```python
from build123d import *

# Parameters (mm, degrees)
F1_DEPTH = 38.1
F2_W     = 31.75
F2_H     = 73.025
F3_DEPTH = 152.401
F4_R     = 2.54
F5_R     = 2.54
F6_R     = 6.35
F7_DEPTH = 25.4
F8_R     = 4.7625
F9_DEPTH = 38.101


with BuildPart() as f1:
    # F0 (on Right) → F1 (new body)
    with BuildSketch(Plane.YZ):
        with BuildLine():
            Line((-57.15, 76.2), (-76.2, 76.2))
            Line((-76.2, 76.2), (-76.2, -13.9112576244))
            Line((-76.2, -13.9112576244), (-50.8, -13.9112576244))
            ThreePointArc((-50.8, -13.9112576244), (-41.275, -23.4362576244), (-50.8, -32.9612576244))
            Line((-50.8, -32.9612576244), (-76.2, -32.9612576244))
            Line((-76.2, -32.9612576244), (-76.2, -76.2))
            Line((-76.2, -76.2), (-38.1, -76.2))
            Line((-38.1, -76.2), (-12.7, -63.5))
            Line((-12.7, -63.5), (-12.7, 19.05))
            Line((-12.7, 19.05), (-57.15, 76.2))
        make_face()
    extrude(amount=F1_DEPTH)

    # F2 (on face) → F3 (cut, through all)
    with BuildSketch(Plane.XY.offset(76.2)):
        with Locations((19.05, -36.5125)):
            Rectangle(F2_W, F2_H)
    extrude(amount=-F3_DEPTH, mode=Mode.SUBTRACT)

    # F4
    f4_edges = [f1.edges().sort_by_distance(p)[0] for p in [
        (3.175, -73.025, 31.144371),
        (34.925, -73.025, 31.144371),
        (34.925, -73.025, -54.580629),
        (3.175, -73.025, -54.580629),
    ]]
    fillet(f4_edges, radius=F4_R)

    # F5
    f5_edges = [f1.edges().sort_by_distance(p)[0] for p in [
        (38.1, -76.2, -54.580629),
        (0, -76.2, -54.580629),
        (0, -76.2, 31.144371),
        (38.1, -76.2, 31.144371),
    ]]
    fillet(f5_edges, radius=F5_R)

    # F6 (on face) → F7 (cut)
    with BuildSketch(Plane.XZ.offset(76.2)):
        with Locations((19.05, -52.0112576244)):
            Circle(F6_R)
    extrude(amount=-F7_DEPTH, mode=Mode.SUBTRACT)

    # F8 (on face) → F9 (cut, through all)
    with BuildSketch(Plane.YZ.offset(38.1)):
        with Locations((-60.96, 57.15)):
            Circle(F8_R)
    extrude(amount=-F9_DEPTH, mode=Mode.SUBTRACT)


solid = f1.part
```
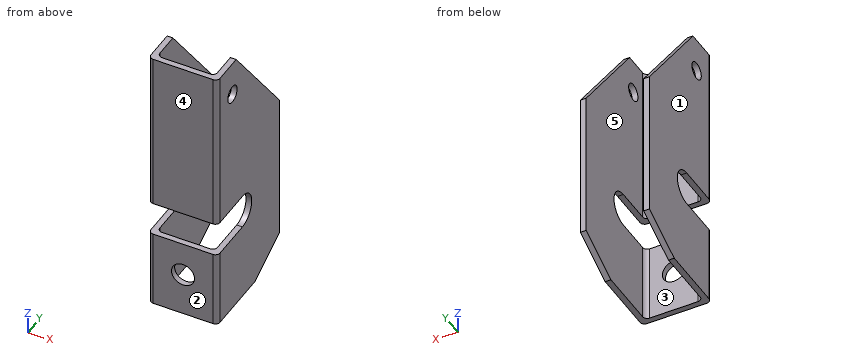
Input: part model. Units: mm. Frame: model coordinates. Face numbers are marked on the shaded views. A direction names the side the tool comes from. Give positions to 0.01 mm unless a question says otherwise; leave off trailing zeros. Order: outer loops, then holes, each group sorted by start corner. A loop starts at its lowest first (then second) coordinate and runs counter-clockwise, first axis right, second up.
1. Cut plane A-A (x = 19.05). Return loops of the section in (y, z) (3 decimals), and give its area (3 significant figures).
Computed:
outline: (-76.2, -76.2) - (-73.025, -76.2) - (-73.025, -58.361) - (-76.2, -58.361) - close; (-76.2, -45.661) - (-73.025, -45.661) - (-73.025, -32.961) - (-76.2, -32.961) - close; (-76.2, -13.911) - (-73.025, -13.911) - (-73.025, 76.2) - (-76.2, 76.2) - close
area: 383 mm2
2. Set-up query: the marked faces 4 and 5. Return all of +Z, -Z, +X, -X, +Y, -Y with unobstructed straight access to the full face (end or side cutting, diameter ignored); none if empty.
Computed:
face 4: +Z, -Z, +X, -X, -Y
face 5: +Z, -Z, +Y
3. Cut plane C-C (z = -54). Return loops of the section in (x, y) (3 decimals).
Computed:
outline: (0, -73.66) arc R2.54 ccw to (2.54, -76.2) - (13.019, -76.2) - (13.019, -73.025) - (5.715, -73.025) arc R2.54 cw to (3.175, -70.485) - (3.175, -12.7) - (0, -12.7) - close; (25.081, -76.2) - (35.56, -76.2) arc R2.54 ccw to (38.1, -73.66) - (38.1, -12.7) - (34.925, -12.7) - (34.925, -70.485) arc R2.54 cw to (32.385, -73.025) - (25.081, -73.025) - close
4. Cut plane B-B (y = -59). Return loops of the section in (x, z) (3 decimals).
Computed:
outline: (0, -76.2) - (3.175, -76.2) - (3.175, -32.961) - (0, -32.961) - close; (0, -13.911) - (3.175, -13.911) - (3.175, 52.81) - (0, 52.81) - close; (0, 61.49) - (3.175, 61.49) - (3.175, 76.2) - (0, 76.2) - close; (34.925, -76.2) - (38.1, -76.2) - (38.1, -32.961) - (34.925, -32.961) - close; (34.925, -13.911) - (38.1, -13.911) - (38.1, 52.81) - (34.925, 52.81) - close; (34.925, 61.49) - (38.1, 61.49) - (38.1, 76.2) - (34.925, 76.2) - close
5. Cut plane D-D (x = 8). Return loops of the section in (y, z) (3 decimals), and give its area (3 significant figures).
Computed:
outline: (-76.2, -76.2) - (-73.025, -76.2) - (-73.025, -32.961) - (-76.2, -32.961) - close; (-76.2, -13.911) - (-73.025, -13.911) - (-73.025, 76.2) - (-76.2, 76.2) - close
area: 423 mm2
6. Draft query along X for the marked faces 1, 2 and 3. Return one class per face: released by +X, released by -X, zero draft, split by the parting line, or undercut.
Computed:
face 1: released by -X
face 2: zero draft
face 3: undercut
7. Pin query (flat end, axial travel): pin 1 Ø8.5 at (y, z) = (-60.96, 57.15) entering from +X; pin 2 Ø8 at (x, z) = (32.5, -18.5) entering from +Y; pin 3 Ø13.5 at (x, z) = (23, -48) entering from +Y (3 decimals). Return the tip coordinate at first contact, or that it passes through.
Computed:
pin 1: passes through
pin 2: stops at y = -12.7
pin 3: stops at y = -73.025
8. Line query: probe 1 along Z at (x, y) = (19.05, -74.8); probe 2 along Z at (x, y) = (36.15, -60.96); probe 3 along X at (y, z) = (-29.5, -11.5) (3 decimals). Output: solid intervals per line, ascending.
Computed:
probe 1: z = -76.2 to -58.36, -45.66 to -32.96, -13.91 to 76.2
probe 2: z = -76.2 to -32.96, -13.91 to 52.39, 61.91 to 76.2
probe 3: x = 0 to 3.175, 34.925 to 38.1
